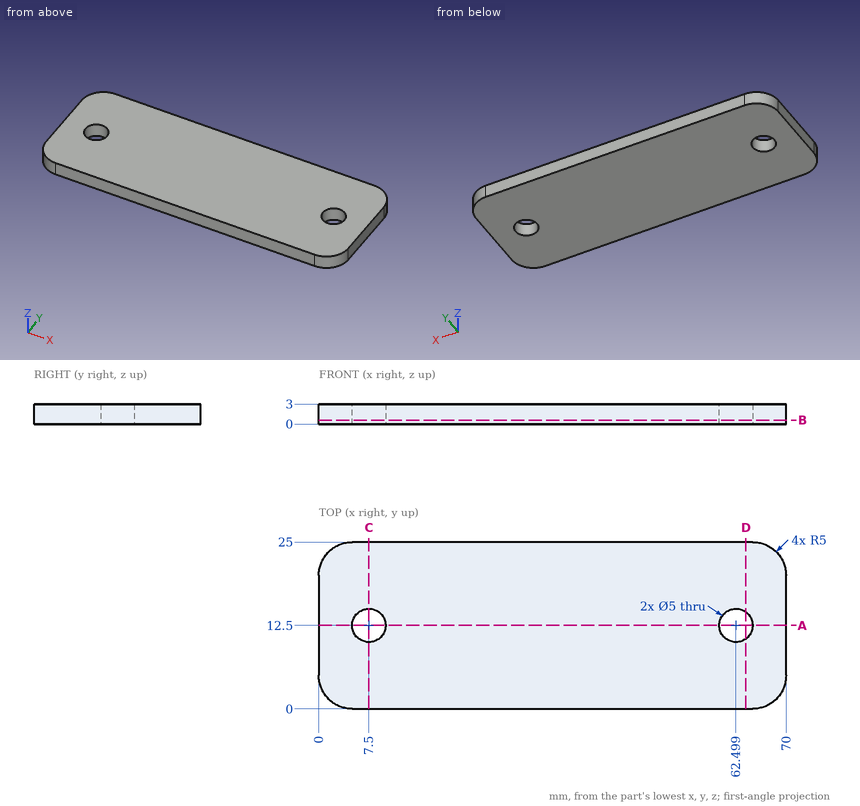
Input: dimensioned drawing with shaded views. Units: mm. Origin: part minimum x, y, z. Round coordinates to 2 decimals unless told otherwise and drop trailing zeros. Loops run counter-clockwise (first coordinate to the right, second up) from the corner with the lowest first, then second, coordinate; pieces in that order, holes last. Notation, with made-up numbers: M 28,35 L 82,35 A26 ccw 82,64 Z; hole C 21,24.25 d6. An arc over 180 degrees is marked long. Return JSON: item names as keys, results as strings. Group by question number.
1. Material intervals for line 1 along Y through (x, z) = (7.5, 1.65); line 2 along X through (y, z) = (12.75, 1.85); line 3 along Y through (x, z) = (63, 1.5), sorted ascending. Write a range as from..to.
2. Section query D-D on x = 64. Output: boundary loops of the cut face in (y, z).
3. Section query C-C on x = 7.5. Output: boundary loops of the cut face in (y, z), and give its area (3 significant figures).
4. Pin query (flat end, axial travel): pin 1 (6.5 mm diameter, centred on x = 7.5, y = 12.5, fed in from +Z). Return the tip coordinate at first contact, or that it passes through.
5. Section query B-B on z = 0.6. Output: boundary loops of the cut face in (x, y).
6. Section query A-A on y = 12.5. Output: boundary loops of the cut face in (x, z).
Checks:
{
 "1": {"line 1": "y = 0..10, 15..25", "line 2": "x = 0..5.01, 9.99..60.01, 64.99..70", "line 3": "y = 0..10.05, 14.95..25"},
 "2": {"outline": "M 0,0 L 10.5,0 L 10.5,3 L 0,3 Z; M 14.5,0 L 25,0 L 25,3 L 14.5,3 Z"},
 "3": {"outline": "M 0,0 L 10,0 L 10,3 L 0,3 Z; M 15,0 L 25,0 L 25,3 L 15,3 Z", "area": "60.0 mm²"},
 "4": {"pin 1": "stops at z = 3"},
 "5": {"outline": "M 0,5 A5 ccw 5,0 L 65,0 A5 ccw 70,5 L 70,20 A5 ccw 65,25 L 5,25 A5 ccw 0,20 Z; hole C 7.5,12.5 d5; hole C 62.5,12.5 d5"},
 "6": {"outline": "M 0,0 L 5,0 L 5,3 L 0,3 Z; M 10,0 L 60,0 L 60,3 L 10,3 Z; M 65,0 L 70,0 L 70,3 L 65,3 Z"}
}
